```python
from build123d import *

# Parameters (mm, degrees)
BOSS_EXTRUDE1_DEPTH = 85
SKETCH4_R           = 30
BOSS_EXTRUDE2_DEPTH = 50
SKETCH5_R           = 22.5
BOSS_EXTRUDE3_DEPTH = 29
SKETCH6_R           = 15
BOSS_EXTRUDE4_DEPTH = 12
BOSS_EXTRUDE5_DEPTH = 75
SKETCH8_R           = 19.5
BOSS_EXTRUDE6_DEPTH = 45
SKETCH9_R           = 11.5
CUT_EXTRUDE1_DEPTH  = 0.1


with BuildPart() as part:
    # Sketch3 → Boss-Extrude1 (new body, symmetric)
    with BuildSketch(Plane(origin=(0, 0, 0), x_dir=(0, 0, -1), z_dir=(1, 0, 0))):
        Polygon((0, 0), (90, 0), (90, 48.125), (18.113318582, 48.125), (0, 56.604840209), (-21.735982298, 10.17580825), align=None)
    extrude(amount=BOSS_EXTRUDE1_DEPTH, both=True)

    # Sketch4 → Boss-Extrude2 (add)
    with BuildSketch(Plane(origin=(0, 48.125, 0), x_dir=(1, 0, 0), z_dir=(0, 1, 0))):
        with Locations((0, 48.113318582)):
            Circle(SKETCH4_R)
    extrude(amount=BOSS_EXTRUDE2_DEPTH)

    # Sketch5 → Boss-Extrude3 (add)
    with BuildSketch(Plane(origin=(0, 98.125, 0), x_dir=(1, 0, 0), z_dir=(0, 1, 0))):
        with Locations((0, 48.113318582)):
            Circle(SKETCH5_R)
    extrude(amount=BOSS_EXTRUDE3_DEPTH)

    # Sketch6 → Boss-Extrude4 (add)
    with BuildSketch(Plane(origin=(0, 127.125, 0), x_dir=(1, 0, 0), z_dir=(0, 1, 0))):
        with Locations((0, 48.113318582)):
            Circle(SKETCH6_R)
    extrude(amount=BOSS_EXTRUDE4_DEPTH)

    # Sketch7 → Boss-Extrude5 (add)
    with BuildSketch(Plane(origin=(0, 10.17580825, 21.735982298), x_dir=(1, 0, 0), z_dir=(0, 0.42399201, 0.905665929))):
        with BuildLine():
            ThreePointArc((-8.058161684, 9.507934936), (0, 7.765075198), (8.058161684, 9.507934936))
            ThreePointArc((8.058161684, 9.507934936), (61.054790967, -7.984924802), (19.407215407, 29.165072602))
            ThreePointArc((19.407215407, 29.165072602), (0, 46.765075198), (-19.407215407, 29.165072602))
            ThreePointArc((-19.407215407, 29.165072602), (-61.054790967, -7.984924802), (-8.058161684, 9.507934936))
        make_face()
    extrude(amount=BOSS_EXTRUDE5_DEPTH)

    # Sketch8 → Boss-Extrude6 (add)
    with BuildSketch(Plane(origin=(0, 41.975209032, 89.660926979), x_dir=(1, 0, 0), z_dir=(0, 0.42399201, 0.905665929))):
        with Locations((-36.373066959, 6.265075198)):
            Circle(SKETCH8_R)
        with Locations((36.373066959, 6.265075198)):
            Circle(SKETCH8_R)
    extrude(amount=BOSS_EXTRUDE6_DEPTH)

    # Sketch9 → Cut-Extrude1 (cut)
    with BuildSketch(Plane(origin=(0, 61.054849502, 130.415893787), x_dir=(1, 0, 0), z_dir=(0, 0.42399201, 0.905665929))):
        with Locations((-36.373066959, 6.265075198)):
            Circle(SKETCH9_R)
        with Locations((36.373066959, 6.265075198)):
            Circle(SKETCH9_R)
    extrude(amount=-CUT_EXTRUDE1_DEPTH, mode=Mode.SUBTRACT)


solid = part.part
```
Design review of the part built by this model. Coordinates are the model's own, in mm. A direction names the side the tool comes from. Round coordinates to 2 decimals unless told otherwise and drop trailing zeros. Order: outer loops, then holes, each group sorted by start corner. A loop starts at its lowest first (then second) coordinate and runs counter-clockwise, first axis right, second up. Notation, with made-up numbers: (-31, 71) - (7, 71) arc R27 ccw to (7, 107) - close; hole circle Ø10 at (75, -11). An arc over 180 degrees is marked (long way). Return JSON: item names as keys, results as strings.
Q1. Machinability: for faces 1 (the flat face through (5, 127.125, -33)), 2 (the cylindrical face through (-61.582, 19.485, 58.204)), 3 (the flat face through (35.984, 2.486, 25.336)), which of the approach directions +Z, -Z, +X, -X, +Y, -Y give a long, thin tool a straight path to every point of the face, cutting with its end or side? Answer none if there is none.
Computed values:
{"face 1": "+Y", "face 2": "none", "face 3": "+X, -X, -Y"}
Q2. For pin 1 Ø21.5 at (x, z) = (21, -64) entering from +Y (3 decimals); pin 2 Ø2 at (x, z) = (47, -19.5) entering from +Y (3 decimals); pin 3 Ø10 at (x, y) = (26.5, 68.5) entering from -Z, all flat-tipped, find the tip position at first contact; note any pin that passes through.
Computed values:
{"pin 1": "stops at y = 127.125", "pin 2": "stops at y = 48.125", "pin 3": "stops at z = -69.04"}
Q3. Consider section D-D on y = 112.5. Write out the cut boundary in (x, z), plus the area to 3 significant figures.
Computed values:
{"outline": "circle Ø45 at (0, -48.11)", "area": "1,590 mm2"}
Q4. Consider section C-C on y = 7. Give the number of separate pieces and of enclosed holes in the cut face, plus the area to 3 significant figures.
Computed values:
{"separate pieces": "3", "enclosed holes": "0", "area": "21,300 mm2"}
Q5. Wall thickness on L1, parallel to Y at x = 48.5, z = -50.5 (3 decimals); L2, parallel to X at y = 22.5, z = 38; L3, parallel to Z at x = -68.5, y = 54: over which ranges is each line inside the solid? List them lowest first. Write a range as [from, to].
Computed values:
{"L1": "y = [0, 48.125]", "L2": "x = [-64.8, -7.94], [7.94, 64.8]", "L3": "z = [-5.56, 1.22]"}
Q6. Consider section B-B on z = -57.5. Write out the cut boundary in (x, y) (3 decimals), plus the area to 3 significant figures.
Computed values:
{"outline": "(-85, 0) - (85, 0) - (85, 48.125) - (28.494, 48.125) - (28.494, 98.125) - (20.448, 98.125) - (20.448, 127.125) - (11.7, 127.125) - (11.7, 139.125) - (-11.7, 139.125) - (-11.7, 127.125) - (-20.448, 127.125) - (-20.448, 98.125) - (-28.494, 98.125) - (-28.494, 48.125) - (-85, 48.125) - close", "area": "12,500 mm2"}
Q7. The part is to be moulded in two halves that separate along Y. For faces 4 (the flat face through (0.12, 13.585, 20.14)), 5 (the flat face through (1, 24, -90)), 6 (the flat face through (36.21, 66.83, 127.6)), say which applies: pulls with the +Y half, pulls with the -Y half, needs draft (parallel to the pull), parting line crosses it, or undercut.
Computed values:
{"face 4": "undercut", "face 5": "needs draft", "face 6": "pulls with the +Y half"}
Q8. Consider section A-A on x = -69. Write out the cut boundary in (y, z) (3 decimals), plus the area to 3 significant figures.
Computed values:
{"outline": "(0, -90) - (48.125, -90) - (48.125, -18.113) - (56.605, 0) - (10.176, 21.736) - (0, 0) - close", "area": "5,020 mm2"}
